The model under review builds one solid part; all positions refer to its coordinate system, in mm. Face numbers are marked on the shaded views. Give positions to 0.01 mm unless a question says otherwise; leave off trailing zeros. Write each loop counter-clockwise with the first axis right and the second up, starting at its lowest first coordinate (ties: lowest second). Pieces come first, ordered by that corner, then holes.
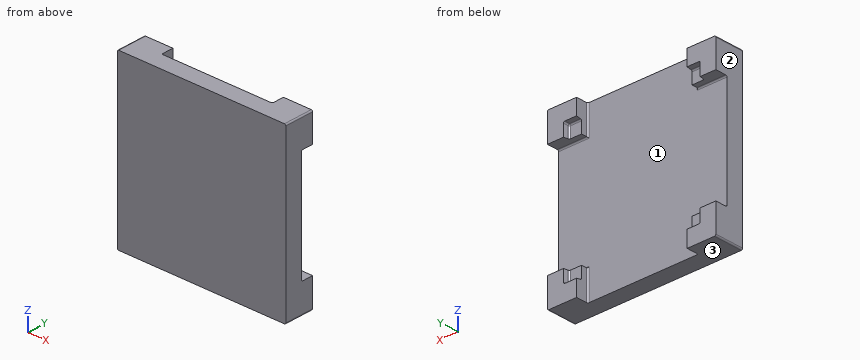
from build123d import *

# Parameters (mm, degrees)
SKETCH1_W           = 125
SKETCH1_H           = 125
BOSS_EXTRUDE1_DEPTH = 21.7
SKETCH2_W           = 100
SKETCH2_H           = 100
CUT_EXTRUDE1_DEPTH  = 9
FILLET2_R           = 1
SKETCH4_W           = 82
SKETCH4_H           = 12.7
SKETCH4_W_2         = 12.3
SKETCH4_H_2         = 82
SKETCH4_H_3         = 12.3
SKETCH4_W_3         = 12.7
CUT_EXTRUDE2_DEPTH  = 9
SKETCH5_W           = 9
SKETCH5_H           = 9
BOSS_EXTRUDE2_DEPTH = 5
DRAFT1_ANGLE        = 10
DRAFT2_ANGLE        = 10
DRAFT3_ANGLE        = 10
DRAFT4_ANGLE        = 10
FILLET3_R           = 1


with BuildPart() as part:
    # Sketch1 → Boss-Extrude1 (new body)
    with BuildSketch(Plane(origin=(0, 0, 0), x_dir=(1, 0, 0), z_dir=(0, 1, 0))):
        with Locations((62.5, 62.5)):
            Rectangle(SKETCH1_W, SKETCH1_H)
    extrude(amount=BOSS_EXTRUDE1_DEPTH)

    # Sketch2 → Cut-Extrude1 (cut)
    with BuildSketch(Plane(origin=(0, 21.7, 0), x_dir=(1, 0, 0), z_dir=(0, 1, 0))):
        with Locations((62.3, 62.3)):
            Rectangle(SKETCH2_W, SKETCH2_H)
    extrude(amount=-CUT_EXTRUDE1_DEPTH, mode=Mode.SUBTRACT)

    # Fillet2
    fillet2_edges = [part.edges().sort_by_distance(p)[0] for p in [
        (0, 10.85, -125),
        (125, 10.85, -125),
        (125, 10.85, 0),
        (0, 10.85, 0),
    ]]
    fillet(fillet2_edges, radius=FILLET2_R)

    # Sketch4 → Cut-Extrude2 (cut)
    with BuildSketch(Plane(origin=(0, 21.7, 0), x_dir=(1, 0, 0), z_dir=(0, 1, 0))):
        with Locations((62.3, 118.65)):
            Rectangle(SKETCH4_W, SKETCH4_H)
        with Locations((6.15, 62.3)):
            Rectangle(SKETCH4_W_2, SKETCH4_H_2)
        with Locations((62.3, 6.15)):
            Rectangle(SKETCH4_W, SKETCH4_H_3)
        with Locations((118.65, 62.3)):
            Rectangle(SKETCH4_W_3, SKETCH4_H_2)
    extrude(amount=-CUT_EXTRUDE2_DEPTH, mode=Mode.SUBTRACT)

    # Sketch5 → Boss-Extrude2 (add)
    with BuildSketch(Plane(origin=(0, 12.7, 0), x_dir=(1, 0, 0), z_dir=(0, 1, 0))):
        with Locations((107.8, 16.8)):
            Rectangle(SKETCH5_W, SKETCH5_H)
        with Locations((16.8, 16.8)):
            Rectangle(SKETCH5_W, SKETCH5_H)
        with Locations((16.8, 107.8)):
            Rectangle(SKETCH5_W, SKETCH5_H)
        with Locations((107.8, 107.8)):
            Rectangle(SKETCH5_W, SKETCH5_H)
    extrude(amount=BOSS_EXTRUDE2_DEPTH)

    # Draft1
    draft1_faces = [part.faces().sort_by_distance(p)[0] for p in [
        (112.3, 19.7, -16.8),
        (107.8, 19.7, -12.3),
    ]]
    draft(draft1_faces, Plane.ZX.offset(17.7), DRAFT1_ANGLE)

    # Draft2
    draft2_faces = [part.faces().sort_by_distance(p)[0] for p in [
        (12.3, 19.7, -16.8),
        (16.8, 19.7, -12.3),
    ]]
    draft(draft2_faces, Plane.ZX.offset(17.7), DRAFT2_ANGLE)

    # Draft3
    draft3_faces = [part.faces().sort_by_distance(p)[0] for p in [
        (16.8, 19.7, -112.3),
        (12.3, 19.7, -107.8),
    ]]
    draft(draft3_faces, Plane.ZX.offset(17.7), DRAFT3_ANGLE)

    # Draft4
    draft4_faces = [part.faces().sort_by_distance(p)[0] for p in [
        (112.3, 19.7, -107.8),
        (107.8, 19.7, -112.3),
    ]]
    draft(draft4_faces, Plane.ZX.offset(17.7), DRAFT4_ANGLE)

    # Fillet3
    fillet3_edges = [part.edges().sort_by_distance(p)[0] for p in [
        (112.652653961, 19.7, -11.947346039),
        (112.3, 17.7, -16.8),
        (107.8, 17.7, -12.3),
        (11.947346039, 19.7, -11.947346039),
        (12.3, 17.7, -16.8),
        (16.8, 17.7, -12.3),
        (11.947346039, 19.7, -112.652653961),
        (12.3, 17.7, -107.8),
        (16.8, 17.7, -112.3),
        (112.652653961, 19.7, -112.652653961),
        (112.3, 17.7, -107.8),
        (107.8, 17.7, -112.3),
        (103.3, 12.7, -114.15),
        (21.3, 12.7, -114.15),
        (10.65, 12.7, -21.3),
        (10.65, 12.7, -103.3),
        (103.3, 12.7, -10.65),
        (21.3, 12.7, -10.65),
        (114.15, 12.7, -21.3),
        (114.15, 12.7, -103.3),
    ]]
    fillet(fillet3_edges, radius=FILLET3_R)


solid = part.part
1) Consider section D-D, the plane z = -86. Give the boundary of the cut face in (x, y), then the cut area to 3 significant figures.
2) The part is to be moulded in two halves that separate along X. For the marked faces 1, 2 and 3, say which applies: +X half, -X half, draft (parallel to the pull), parting line (faces both ways), or undercut.
3) To check wall thickness, follow probe 1 along Z at (x, y) = (109.5, 16); probe 2 along Y at (x, z) = (48.5, -22). State the ranges of each line that lie inside material, in increasing order.
4) Insertion check: pin 1 (2 mm diameter, centred on y = 15.5, z = -43, fed in from -X); pin 2 (4 mm diameter, centred on x = 109.5, z = -16, fed in from +Y); pin 3 (4 mm diameter, centred on x = 81, z = -65.5, fed in from +Y). Each pin has a flat end and moves straight along its axis. Give the tip position at first contact, or say it passes through.
5) Consider section C-C, the plane x = 83.5. Give the boundary of the cut face in (y, z).
6) Consider section B-B, the plane z = -10. Give the boundary of the cut face in (x, y).
7) Consider section A-A, the plane y = 15.25. Give the boundary of the cut face in (x, z), then the cut area to 3 significant figures.
Answer block:
1. outline: (0, 0) - (125, 0) - (125, 12.7) - (0, 12.7) - close
1. area: 1,590 mm2
2. face 1: undercut
2. face 2: -X half
2. face 3: draft
3. probe 1: z = -125 to -103.3, -21.3 to 0
3. probe 2: y = 0 to 12.7
4. pin 1: passes through
4. pin 2: stops at y = 17.7
4. pin 3: stops at y = 12.7
5. outline: (0, -125) - (12.7, -125) - (12.7, 0) - (0, 0) - close
6. outline: (0, 0) - (125, 0) - (125, 21.7) - (103.3, 21.7) - (103.3, 13.7) arc R1 cw to (102.3, 12.7) - (22.3, 12.7) arc R1 cw to (21.3, 13.7) - (21.3, 21.7) - (0, 21.7) - close
7. outline: (0, -124) arc R1 ccw to (1, -125) - (21.3, -125) - (21.3, -103.3) - (0, -103.3) - close; (0, -21.3) - (21.3, -21.3) - (21.3, 0) - (1, 0) arc R1 ccw to (0, -1) - close; (103.3, -125) - (124, -125) arc R1 ccw to (125, -124) - (125, -103.3) - (103.3, -103.3) - close; (103.3, -21.3) - (125, -21.3) - (125, -1) arc R1 ccw to (124, 0) - (103.3, 0) - close
7. area: 1,850 mm2
